CAD build for the part. Positions are in the model's coordinates, mm. A direction names the side the tool comes from. Give positions to 0.01 mm unless a question says otherwise; leave off trailing zeros. Loops run counter-clockwise (first coordinate to the right, second up) from the corner with the lowest first, then second, coordinate; pieces in that order, holes last. Notation, with made-up numbers: (-16, -12.75) -> (-9, -12.75) arc R9 cw to (-9, 4.25) -> close; hole circle Ø8 at (48, -6). An arc over 180 degrees is marked (long way). Use one line per item in the form item = value.
```python
from build123d import *

# Parameters (mm, degrees)
SKETCH_W           = 20
SKETCH_H           = 11
PAD_DEPTH          = 21
SKETCH001_W        = 20
SKETCH001_H        = 5
PAD001_DEPTH       = 8
SKETCH002_W        = 6.4
SKETCH002_H        = 9.70104
POCKET_DEPTH       = 16
SKETCH003_W        = 4
SKETCH003_H        = 2.091244
POCKET001_DEPTH    = 16
SKETCH005_R        = 2.7
POCKET002_DEPTH    = 3
SKETCH006_R        = 1.7
POCKET003_DEPTH    = 15
PAD002_DEPTH       = 1
PAD003_DEPTH       = 1
PAD004_DEPTH       = 8
PAD005_DEPTH       = 8
PAD006_DEPTH       = 1
PAD007_DEPTH       = 1
PAD007_FACE27_W    = 9
PAD007_FACE27_H    = 14
PAD008_DEPTH       = 0.1
PAD008_FACE24_W    = 9
PAD008_FACE24_H    = 14
PAD009_DEPTH       = 0.1
SKETCH009_W        = 11.765216
SKETCH009_H        = 12.105414
POCKET007_DEPTH    = 23
SKETCH010_W        = 8
SKETCH010_H        = 5
PAD010_DEPTH       = 6
PAD011_DEPTH       = 25
SKETCH012_W        = 7.888134
SKETCH012_H        = 1
PAD012_DEPTH       = 23
SKETCH014_R        = 2
POCKET008_DEPTH    = 5
SKETCH016_W        = 9.43169
SKETCH016_H        = 30.019524
POCKET010_DEPTH    = 5
SKETCH019_W        = 10.102889
SKETCH019_H        = 7.195522
POCKET012_DEPTH    = 6
SKETCH020_R        = 4.8264255923
POCKET014_DEPTH    = 0.5
POCKET015_DEPTH    = 2
COPYSKETCH024_R    = 1.1
POCKET017_DEPTH    = 3
SKETCH025_R        = 1.7
POCKET018_DEPTH    = 1
SKETCH026_R        = 2.010288662
POCKET019_DEPTH    = 5
COPYSKETCH027_R    = 2.99206
POCKET020_DEPTH    = 0.5
COPYSKETCH027001_W = 6.010766
COPYSKETCH027001_H = 4.360142
POCKET021_DEPTH    = 25


with BuildPart() as part:
    # Sketch → Pad (new body)
    with BuildSketch(Plane.XY):
        Rectangle(SKETCH_W, SKETCH_H)
    extrude(amount=PAD_DEPTH)

    # Sketch001 (on Face1 of Pad) → Pad001 (join)
    with BuildSketch(Plane.XZ.offset(5.5)):
        with Locations((0, 2.5)):
            Rectangle(SKETCH001_W, SKETCH001_H)
    extrude(amount=PAD001_DEPTH)

    # Sketch002 (on Face4 of Pad001) → Pocket (cut)
    with BuildSketch(Plane.XY.offset(21)):
        with Locations((0, 1.35052)):
            Rectangle(SKETCH002_W, SKETCH002_H)
    extrude(amount=-POCKET_DEPTH, mode=Mode.SUBTRACT)

    # Sketch003 (on Face4 of Pocket) → Pocket001 (cut)
    with BuildSketch(Plane.XY.offset(21)):
        with Locations((0, -4.482633)):
            Rectangle(SKETCH003_W, SKETCH003_H)
    extrude(amount=-POCKET001_DEPTH, mode=Mode.SUBTRACT)

    # Sketch005 (on Face5 of Pocket001) → Pocket002 (cut)
    with BuildSketch(Plane.XY.offset(5)):
        with Locations((0, -9.4740693718)):
            Circle(SKETCH005_R)
    extrude(amount=-POCKET002_DEPTH, mode=Mode.SUBTRACT)

    # Sketch006 (on Face24 of Pocket002) → Pocket003 (cut)
    with BuildSketch(Plane.XY.offset(2)):
        with Locations((0, -9.4740693718)):
            Circle(SKETCH006_R)
    extrude(amount=-POCKET003_DEPTH, mode=Mode.SUBTRACT)

    # Pocket003 Face21 → Pad002 (add)
    with BuildSketch(Plane(origin=(0, 1.0196321739, 5), x_dir=(0, 1, 0), z_dir=(0, 0, 1))):
        Polygon((4.4803678261, -3.2), (4.4803678261, 3.2), (-4.5196321739, 3.2), (-4.5196321739, 2), (-4.4566431739, 2), (-4.4566431739, -2), (-4.5196321739, -2), (-4.5196321739, -3.2), align=None)
    extrude(amount=PAD002_DEPTH)

    # Pad002 Face3 → Pad003 (add)
    with BuildSketch(Plane(origin=(6.4756476684, -0.1398963731, 21), x_dir=(0, 1, 0), z_dir=(0, 0, 1))):
        Polygon((-3.3601036269, 4.4756476684), (-5.3601036269, 4.4756476684), (-5.3601036269, -3.5243523316), (5.6398963731, -3.5243523316), (5.6398963731, 3.2756476684), (-3.3601036269, 3.2756476684), align=None)
    extrude(amount=PAD003_DEPTH)

    # Pad003 Face22 → Pad004 (add)
    with BuildSketch(Plane(origin=(-6.4756476684, -0.1398963731, 21), x_dir=(0, 1, 0), z_dir=(0, 0, 1))):
        Polygon((5.6398963731, -3.2756476684), (5.6398963731, 3.5243523316), (-5.3601036269, 3.5243523316), (-5.3601036269, -4.4756476684), (-3.3601036269, -4.4756476684), (-3.3601036269, -3.2756476684), align=None)
    extrude(amount=PAD004_DEPTH)

    # Pad004 Face11 → Pad005 (add)
    with BuildSketch(Plane(origin=(6.4756476684, -0.1398963731, 22), x_dir=(0, 1, 0), z_dir=(0, 0, 1))):
        Polygon((-3.3601036269, 4.4756476684), (-5.3601036269, 4.4756476684), (-5.3601036269, -3.5243523316), (5.6398963731, -3.5243523316), (5.6398963731, 3.2756476684), (-3.3601036269, 3.2756476684), align=None)
    extrude(amount=PAD005_DEPTH)

    # Pad005 Face40 → Pad006 (add)
    with BuildSketch(Plane(origin=(-6.4756476684, -0.1398963731, 29), x_dir=(0, 1, 0), z_dir=(0, 0, 1))):
        Polygon((5.6398963731, -3.2756476684), (5.6398963731, 3.5243523316), (-5.3601036269, 3.5243523316), (-5.3601036269, -4.4756476684), (-3.3601036269, -4.4756476684), (-3.3601036269, -3.2756476684), align=None)
    extrude(amount=PAD006_DEPTH)

    # Pad006 Face33 → Pad007 (add)
    with BuildSketch(Plane(origin=(0, 1.0196321739, 6), x_dir=(0, 1, 0), z_dir=(0, 0, 1))):
        Polygon((4.4803678261, -3.2), (4.4803678261, 3.2), (-4.5196321739, 3.2), (-4.5196321739, 2), (-4.4566431739, 2), (-4.4566431739, -2), (-4.5196321739, -2), (-4.5196321739, -3.2), align=None)
    extrude(amount=PAD007_DEPTH)

    # Pad007 Face27 → Pad008 (add)
    with BuildSketch(Plane(origin=(3.2, 1, 14), x_dir=(0, 1, 0), z_dir=(-1, 0, 0))):
        Rectangle(PAD007_FACE27_W, PAD007_FACE27_H)
    extrude(amount=PAD008_DEPTH)

    # Pad008 Face24 → Pad009 (add)
    with BuildSketch(Plane(origin=(-3.2, 1, 14), x_dir=(0, -1, 0), z_dir=(1, 0, 0))):
        Rectangle(PAD008_FACE24_W, PAD008_FACE24_H)
    extrude(amount=PAD009_DEPTH)

    # Sketch009 → Pocket007 (cut)
    with BuildSketch(Plane.XY.offset(30)):
        with Locations((7.044694, 0.235483)):
            Rectangle(SKETCH009_W, SKETCH009_H)
    extrude(amount=-POCKET007_DEPTH, mode=Mode.SUBTRACT)

    # Sketch010 → Pad010 (join)
    with BuildSketch(Plane(origin=(-4, 0, 0), x_dir=(0, -1, 0), z_dir=(-1, 0, 0))):
        with Locations((9.5, 2.5)):
            Rectangle(SKETCH010_W, SKETCH010_H)
    extrude(amount=PAD010_DEPTH)

    # Sketch011 (on Face16 of Pad010) → Pad011 (join)
    with BuildSketch(Plane.XY.offset(5)):
        Polygon((-5.0802496781, -5.4306888829), (-5.170571, -13.486972), (10.046902, -13.556283), (9.9827916781, -5.539257), (8.9827916781, -5.527363), (8.9827916781, -12.430687), (-4.0802496781, -12.430687), (-4.0802496781, -5.4306871171), align=None)
    extrude(amount=PAD011_DEPTH)

    # Sketch012 (on Face3 of Pad011) → Pad012 (join)
    with BuildSketch(Plane.XY.offset(7)):
        with Locations((6.031892, -4.9664883219)):
            Rectangle(SKETCH012_W, SKETCH012_H)
    extrude(amount=PAD012_DEPTH)

    # Sketch014 (on Face24 of Pad012) → Pocket008 (cut)
    with BuildSketch(Plane(origin=(9.9378599981, 0.0794707917, 0), x_dir=(-0.0079965154, 0.9999680274, 0), z_dir=(0.9999680274, 0.0079965154, 0))):
        with Locations((-9.393911, 10.196385)):
            Circle(SKETCH014_R)
    extrude(amount=-POCKET008_DEPTH, mode=Mode.SUBTRACT)

    # Sketch016 → Pocket010 (cut)
    with BuildSketch(Plane(origin=(-10, 0, 0), x_dir=(0, -1, 0), z_dir=(-1, 0, 0))):
        with Locations((-1.020089, 15.009762)):
            Rectangle(SKETCH016_W, SKETCH016_H)
    extrude(amount=-POCKET010_DEPTH, mode=Mode.SUBTRACT)

    # Sketch019 → Pocket012 (cut)
    with BuildSketch(Plane.YZ.offset(10)):
        with Locations((0.5744515, 3.409147)):
            Rectangle(SKETCH019_W, SKETCH019_H)
    extrude(amount=-POCKET012_DEPTH, mode=Mode.SUBTRACT)

    # Sketch020 → Pocket014 (cut)
    with BuildSketch(Plane.XY.offset(2)):
        with Locations((-0.021918, 17.928259)):
            Circle(SKETCH020_R)
    extrude(amount=-POCKET014_DEPTH, mode=Mode.SUBTRACT)

    # Sketch022 (on Face189 of Pocket014) → Pocket015 (cut)
    with BuildSketch(Plane.XY.offset(2)):
        with BuildLine():
            add(Edge.make_bspline(
                [(-1.975646, 22.546564), (-3.685938, 22.005808), (-4.331799, 20.570465)],
                knots=[0, 0, 0, 1, 1, 1], degree=2))
            Line((-4.331799, 20.570465), (-4.136705, 22.627766))
            Line((-4.136705, 22.627766), (-1.975646, 22.546564))
        make_face()
    extrude(amount=-POCKET015_DEPTH, mode=Mode.SUBTRACT)

    # CopySketch024 → Pocket017 (cut)
    with BuildSketch(Plane(origin=(-5, 0, 0), x_dir=(0, -1, 0), z_dir=(-1, 0, 0))):
        with Locations((0, 12)):
            Circle(COPYSKETCH024_R)
        with Locations((0, 20.5)):
            Circle(COPYSKETCH024_R)
    extrude(amount=-POCKET017_DEPTH, mode=Mode.SUBTRACT)

    # Sketch025 (on Face29 of Pocket017) → Pocket018 (cut)
    with BuildSketch(Plane(origin=(-5, 0, 0), x_dir=(0, -1, 0), z_dir=(-1, 0, 0))):
        with Locations((0, 20.5)):
            Circle(SKETCH025_R)
        with Locations((0, 12)):
            Circle(SKETCH025_R)
    extrude(amount=-POCKET018_DEPTH, mode=Mode.SUBTRACT)

    # Sketch026 (on Face48 of Pocket018) → Pocket019 (cut)
    with BuildSketch(Plane(origin=(-0.0615350782, -13.5102421178, 0), x_dir=(0.9999896275, -0.0045546512, 0), z_dir=(-0.0045546512, -0.9999896275, 0))):
        with Locations((0, 20.130779)):
            Circle(SKETCH026_R)
        with BuildLine():
            add(Edge.make_bspline(
                [(3.15934, 18.981977), (2.637434, 17.541506), (1.323444, 16.977846)],
                knots=[0, 0, 0, 1, 1, 1], degree=2))
            Line((1.323444, 16.977846), (1.323444, 10.931852))
            add(Edge.make_bspline(
                [(3.15934, 13.575), (1.886149, 14.090854), (1.323444, 10.931852)],
                knots=[0, 0, 0, 1, 1, 1], degree=2))
            Line((3.15934, 13.575), (3.15934, 18.981977))
        make_face()
        with BuildLine():
            add(Edge.make_bspline(
                [(-2.481979, 22.206863), (-2.206434, 23.233652), (-0.682459, 23.421541)],
                knots=[0, 0, 0, 1, 1, 1], degree=2))
            Line((-0.682459, 23.421541), (-2.210586, 23.939598))
            Line((-2.210586, 23.939598), (-2.481979, 22.206863))
        make_face()
    extrude(amount=-POCKET019_DEPTH, mode=Mode.SUBTRACT)

    # CopySketch027 → Pocket020 (cut)
    with BuildSketch(Plane.XZ.offset(13.5)):
        with Locations((0, 20.130779)):
            Circle(COPYSKETCH027_R)
    extrude(amount=-POCKET020_DEPTH, mode=Mode.SUBTRACT)

    # CopySketch027001 → Pocket021 (cut)
    with BuildSketch(Plane.XY.offset(30)):
        with Locations((-8.005399, -4.370609)):
            Rectangle(COPYSKETCH027001_W, COPYSKETCH027001_H)
    extrude(amount=-POCKET021_DEPTH, mode=Mode.SUBTRACT)


solid = part.part
```
1. Cut at A-A, the plane y = 0. Write the cut outline in (x, z), then the cut area to 3 significant figures.
Result sheet:
outline = (-5, 0) -> (4, 0) -> (4, 7) -> (-3.1, 7) -> (-3.1, 10.9) -> (-4, 10.9) -> (-4, 10.3) -> (-5, 10.3) -> close; (-5, 13.7) -> (-4, 13.7) -> (-4, 13.1) -> (-3.1, 13.1) -> (-3.1, 19.4) -> (-4, 19.4) -> (-4, 18.8) -> (-5, 18.8) -> close; (-5, 22.2) -> (-4, 22.2) -> (-4, 21.6) -> (-3.2, 21.6) -> (-3.2, 30) -> (-5, 30) -> close
area = 95.1 mm^2
2. Drill centre lines: line 1 (Z direction, x = -3.55, y = 0); line 2 (Y direction, x = -3.25, z = 20.5); line 3 (Z direction, x = 0, y = -13.2). Where is each one in solid material? Low to high.
Result sheet:
line_1 = 0 to 10.9, 13.1 to 19.4, 21.6 to 30
line_2 = -13.5 to -12.43, -5.5 to -1.1, 1.1 to 5.5
line_3 = 0 to 17.14, 23.12 to 30
3. Tool access for faces 4 (the cylindrical face through (-4.507, 0.221, 22.186)), 5 (the flat face through (-3, -5.5, 17)), 6 (the flat face through (2, -4, 6)), 7 (the cylindrical face through (-3.556, 0.238, 19.426)), 8 (the flat face through (2.088, -5, 18)): list every direction of +Z, -Z, +X, -X, +Y, -Y with a clear straight run to the whole face (end or side of a thin tool).
Result sheet:
face_4 = -X
face_5 = +Z, +X
face_6 = +Z
face_7 = +X, -X
face_8 = +Z, +Y
4. Mould opens along Y. For faces 1 (the flat face through (2, -13, 21)), 2 (the flat face through (9.976, -5, 18)), 3 (the flat face through (7, -4.477, 3)) say: pulls with the +Y half, pulls with the -Y half, needs draft (parallel to the pull), parting line crosses it, or undercut.
Result sheet:
face_1 = undercut
face_2 = needs draft
face_3 = pulls with the +Y half
5. Cut at D-D, the plane x = 0. State how many separate pieces and enclosed holes the cut face has, then the cut area to 3 significant figures.
Result sheet:
separate_pieces = 3
enclosed_holes = 0
area = 112 mm^2
6. Drop flat-ended pins along their axis: P1, Ø2.5, axis at x = -2.5, z = 3, coming from the -Y side; P2, Ø3, axis at y = -9.5, z = 13, coming from the +X side; P3, Ø5.5, axis at x = -7, z = 15.5, coming from the +Y side; P4, Ø5.5, axis at y = 2.5, z = 3.5, coming from the +X side. Give the stop position or say it passes through.
Result sheet:
P1 = -13.5
P2 = 10.03
P3 = 5.5
P4 = 4
7. Cut at C-C, the plane y = 2.75. Write the cut outline in (x, z).
Result sheet:
outline = (-5, 0) -> (4, 0) -> (4, 7) -> (-3.1, 7) -> (-3.1, 21) -> (-3.2, 21) -> (-3.2, 30) -> (-5, 30) -> close
